Autodesk Fusion 360 part; units mm, degrees
sketch "Sketch1" plane through (0, 0, 0) normal (0, 0, 1) x (1, 0, 0)
  line L0 (0, 0) -> (-170, 0)
  line L1 (-170, 0) -> (-170, -80)
  line L2 (-170, -80) -> (0, -80)
  line L3 (0, -80) -> (0, 0)
  dimension "d1" = 170
  dimension "d2" = 80
extrude "Extrude1" add sketch "Sketch1" along normal blind 30
sketch "Sketch2" plane through (0, 0, 30) normal (0, 0, 1) x (-1, 0, 0)
  line L0 (0, 80) -> (0, 0)
  line L1 (0, 0) -> (170, 0)
  line L2 (170, 0) -> (170, 80)
  line L3 (170, 80) -> (0, 80)
  line L4 (0, 80) -> (40, 80)
  line L5 (40, 80) -> (40, 0)
  line L6 (40, 0) -> (0, 0)
  line L7 (0, 0) -> (0, 80)
  dimension "d5" = 40
extrude "Extrude2" add sketch "Sketch2" along normal blind 50 contours L0 L1 L3 L4 L5 L6 L7
sketch "Sketch3" plane through (0, 0, 80) normal (0, 0, 1) x (-1, 0, 0)
  line L0 (0, 0) -> (40, 0)
  line L1 (40, 0) -> (40, 80)
  line L2 (40, 80) -> (0, 80)
  line L3 (0, 80) -> (0, 0)
  line L4 (0, 80) -> (10, 80)
  line L5 (10, 80) -> (10, 0)
  line L6 (10, 0) -> (0, 0)
  line L7 (0, 0) -> (0, 80)
extrude "Extrude3" cut sketch "Sketch3" along normal blind 0 and the other way blind 30 contours L0 L2 L3 L4 L5 L6 L7
fillet "Fillet1" radius 30 1 edges at (-10, -40, 80)
sketch "Sketch4" plane through (0, 0, 30) normal (0, 0, 1) x (-1, 0, 0)
  line L0 (40, 80) -> (40, 0)
  line L1 (40, 0) -> (170, 0)
  line L2 (170, 0) -> (170, 80)
  line L3 (170, 80) -> (40, 80)
  line L4 (170, 80) -> (140, 80)
  line L5 (140, 80) -> (140, 0)
  line L6 (140, 0) -> (170, 0)
  line L7 (170, 0) -> (170, 80)
extrude "Extrude4" add sketch "Sketch4" along normal blind 20 contours L1 L2 L3 L4 L5 L6 L7
sketch "Sketch5" plane through (-170, 0, 0) normal (-1, 0, 0) x (0, -1, 0)
  line L0 (0, 0) -> (80, 0)
  line L1 (80, 0) -> (80, 50)
  line L2 (80, 50) -> (0, 50)
  line L3 (0, 50) -> (0, 0)
  circle A0 centre (40, 50) radius 20
  dimension "d16" = 40
extrude "Extrude5" add sketch "Sketch5" along normal blind 0 and the other way blind 30 contours L2 A0 picked at (45.5083, 53.7555)
sketch "Sketch6" plane through (0, 0, 30) normal (0, 0, 1) x (-1, 0, 0)
  line L0 (140, 0) -> (140, 80)
  line L1 (140, 80) -> (40, 80)
  line L2 (40, 80) -> (40, 0)
  line L3 (40, 0) -> (140, 0)
  line L4 (140, 50) -> (40, 50)
  line L5 (40, 50) -> (40, 30)
  line L6 (40, 30) -> (140, 30)
  line L7 (140, 30) -> (140, 50)
extrude "Extrude6" add sketch "Sketch6" along normal blind 10 contours L0 L2 L4 L5 L6 L7
sketch "Sketch7" plane through (0, 0, 0) normal (1, 0, 0) x (0, 1, 0)
  line L0 (0, 50) -> (-80, 50)
  line L1 (-80, 50) -> (-80, 0)
  line L2 (-80, 0) -> (0, 0)
  line L3 (0, 0) -> (0, 50)
  line L4 (-60, 0) -> (-20, 0)
  line L5 (-20, 0) -> (-20, 20)
  line L6 (-20, 20) -> (-60, 20)
  line L7 (-60, 20) -> (-60, 0)
  line L8 (-50, 20) -> (-30, 20)
  line L9 (-30, 20) -> (-30, 40)
  line L10 (-30, 40) -> (-50, 40)
  line L11 (-50, 40) -> (-50, 20)
extrude "Extrude7" cut sketch "Sketch7" along normal blind 0 and the other way blind 170 contours L2 L4 L5 L6 L7 L8 | L6 L8 L9 L10 L11
sketch "Sketch8" plane through (0, 0, 30) normal (0, 0, 1) x (-1, 0, 0)
  line L0 (140, 30) -> (40, 30)
  line L1 (40, 30) -> (40, 0)
  line L2 (40, 0) -> (140, 0)
  line L3 (140, 0) -> (140, 30)
  line L4 (40, 30) -> (140, 30)
  line L5 (140, 30) -> (140, 29)
  line L6 (140, 29) -> (40, 29)
  line L7 (40, 29) -> (40, 30)
  line L8 (40, 50) -> (140, 50)
  line L9 (140, 50) -> (140, 51)
  line L10 (140, 51) -> (40, 51)
  line L11 (40, 51) -> (40, 50)
  dimension "d27" = 1
  dimension "d28" = 100
  dimension "d29" = 1
extrude "Extrude8" add sketch "Sketch8" along normal blind 10 contours L0 L1 L3 L4 L5 L6 L7 | L8 L9 L10 L11
sketch "Sketch9" plane through (0, 0, 40) normal (0, 0, 1) x (-1, 0, 0)
  line L0 (40, 29) -> (140, 29)
  line L1 (140, 29) -> (140, 30)
  line L2 (140, 30) -> (40, 30)
  line L3 (40, 30) -> (40, 29)
  line L4 (40, 51) -> (140, 51)
  line L5 (140, 51) -> (140, 29)
  line L6 (140, 29) -> (40, 29)
  line L7 (40, 29) -> (40, 51)
extrude "Extrude9" add sketch "Sketch9" along normal blind 1
Model file for the job. Use its own axes, mm. A direction names the side the tool comes from. Give positions to 0.01 mm unless a question says otherwise; leave off trailing zeros. Loops run counter-clockwise (first coordinate to the right, second up) from the corner with the lowest first, then second, coordinate; pieces in that order, holes last. Notation, with made-up numbers: (5.5, 39) -> (20.5, 39) arc R16 cw to (20.5, 70) -> close; hole circle Ø5 at (71, -3). An arc over 180 degrees is marked (long way). Use a Markdown table: item, result. Add a question column.
(1) Wall check: line 1 along Y through (x, z) = (-33, 27.5); line 2 along Y through (x, z) = (-117.5, 15); line 3 along X through (y, z) = (-9.5, 35.5). Give the ranges that are in metal, low to high.
(2) Slice it at C-C on x = -55. List the corners of the cut face in (y, z).
(3) Slice it at D-D on z = 62.5. List the corners of the cut face in (x, y), and give its area (3 significant figures).
(4) Mould opens along Y. For faces 6 (the flat face through (-84, 0, 22)), 7 (the flat face through (-84, -40, 40)), 8 (the flat face through (-5, -41, 50)) say: +Y half, -Y half, draft (parallel to the pull), parting line (faces both ways), or undercut.
(5) Drop flat-ended pins along their axis: pin 1 Ø9 at (x, z) = (-78, 34) entering from -Y; pin 2 Ø1.5 at (x, y) = (-67.5, -62) entering from +Z; pin 3 Ø2 at (x, y) = (-74, -21.5) entering from -Z; pin 4 Ø4 at (x, y) = (-150, -16.5) entering from +Z. Give the stop position or say it passes through.
(6) Slice it at A-A on z = 46. List the corners of the cut face in (x, y), and give its area (3 significant figures).
(7) Tool access for faces 1 (the flat face through (-91, -65, 30)), 2 (the flat face through (-89, -40, 41)), 3 (the flat face through (-91, -14, 30)), 4 (the flat face through (-84, -20, 10)), 5 (the flat face through (-155, -70, 50)): list every direction of +Z, -Z, +X, -X, +Y, -Y with a clear straight run to the whole face (end or side of a thin tool).
Filled sheet:
| question | item | result |
|---|---|---|
| 1 | line 1 | -80 to -50, -30 to 0 |
| 1 | line 2 | -80 to -60, -20 to 0 |
| 1 | line 3 | -170 to -140, -40 to 0 |
| 2 | outline | (-80, 0) -> (-60, 0) -> (-60, 20) -> (-50, 20) -> (-50, 40) -> (-30, 40) -> (-30, 20) -> (-20, 20) -> (-20, 0) -> (0, 0) -> (0, 30) -> (-29, 30) -> (-29, 41) -> (-51, 41) -> (-51, 30) -> (-80, 30) -> close |
| 3 | outline | (-170, -55.61) -> (-140, -55.61) -> (-140, -24.39) -> (-170, -24.39) -> close; (-40, -80) -> (-12.73, -80) -> (-12.73, 0) -> (-40, 0) -> close |
| 3 | area | 3,120 mm2 |
| 4 | face 6 | +Y half |
| 4 | face 7 | undercut |
| 4 | face 8 | draft |
| 5 | pin 1 | y = -80 |
| 5 | pin 2 | z = 30 |
| 5 | pin 3 | z = 20 |
| 5 | pin 4 | z = 50 |
| 6 | outline | (-170, -80) -> (-140, -80) -> (-140, 0) -> (-170, 0) -> close; (-40, -80) -> (0, -80) -> (0, 0) -> (-40, 0) -> close |
| 6 | area | 5,600 mm2 |
| 7 | face 1 | +Z, -Y |
| 7 | face 2 | +Z, +Y, -Y |
| 7 | face 3 | +Z, +Y |
| 7 | face 4 | -Z, +X, -X |
| 7 | face 5 | +Z, -X, -Y |
